from build123d import *

# Parameters (mm, degrees)
SKETCH2_W               = 121
SKETCH2_H               = 180
BOSS_EXTRUDE1_DEPTH     = 970
CUT_EXTRUDE1_DEPTH      = 1359.721825835
CUT_EXTRUDE1_DEPTH_BACK = 1359.721825835
CUT_EXTRUDE5_DEPTH      = 1625
SKETCH4_R               = 8.5
CUT_EXTRUDE6_DEPTH      = 78


with BuildPart() as part:
    # Sketch2 → Boss-Extrude1 (new body)
    with BuildSketch(Plane(origin=(0, 0, 0), x_dir=(1, 0, 0), z_dir=(0, 1, 0))):
        Polygon((300, -515), (800, -515), (800, 515), (300, 515), (300, 175), (-404, 175), (-525, 175), (-800, 175), (-800, -175), (300, -175), align=None)
        with Locations((-464.5, 265)):
            Rectangle(SKETCH2_W, SKETCH2_H)
    extrude(amount=BOSS_EXTRUDE1_DEPTH)

    # Sketch1 → Cut-Extrude1 (cut, two sides: drawn at the far end of the back side and taken through both)
    with BuildSketch(Plane.XY.offset(-CUT_EXTRUDE1_DEPTH_BACK)):
        Polygon((-800, 970), (530, 970), (300, 730), (-400, 600), (-800, 500), align=None)
    extrude(amount=CUT_EXTRUDE1_DEPTH + CUT_EXTRUDE1_DEPTH_BACK, mode=Mode.SUBTRACT)

    # Sketch3 → Cut-Extrude5 (cut)
    with BuildSketch(Plane.ZY.offset(800)):
        with BuildLine():
            Line((-165, 100), (-165, 20))
            ThreePointArc((-165, 20), (-162.071067812, 12.928932188), (-155, 10))
            Line((-155, 10), (-75, 10))
            ThreePointArc((-75, 10), (-67.928932188, 12.928932188), (-65, 20))
            Line((-65, 20), (-65, 100))
            ThreePointArc((-65, 100), (-67.928932188, 107.071067812), (-75, 110))
            Line((-75, 110), (-155, 110))
            ThreePointArc((-155, 110), (-162.071067812, 107.071067812), (-165, 100))
        make_face()
        with BuildLine():
            Line((75, 110), (155, 110))
            ThreePointArc((155, 110), (162.071067812, 107.071067812), (165, 100))
            Line((165, 100), (165, 20))
            ThreePointArc((165, 20), (162.071067812, 12.928932188), (155, 10))
            Line((155, 10), (75, 10))
            ThreePointArc((75, 10), (67.928932188, 12.928932188), (65, 20))
            Line((65, 20), (65, 100))
            ThreePointArc((65, 100), (67.928932188, 107.071067812), (75, 110))
        make_face()
    extrude(amount=-CUT_EXTRUDE5_DEPTH, mode=Mode.SUBTRACT)

    # Sketch4 → Cut-Extrude6 (cut)
    with BuildSketch(Plane.XZ):
        with Locations(Location((-498.5, 115, 0), (0, 0, 270))):
            Circle(SKETCH4_R)
        with Locations(Location((-501, -115, 0), (0, 0, 270))):
            Circle(SKETCH4_R)
        with Locations(Location((501, -115, 0), (0, 0, 270))):
            Circle(SKETCH4_R)
        with Locations(Location((498.5, 115, 0), (0, 0, 90))):
            Circle(SKETCH4_R)
    extrude(amount=-CUT_EXTRUDE6_DEPTH, mode=Mode.SUBTRACT)


solid = part.part
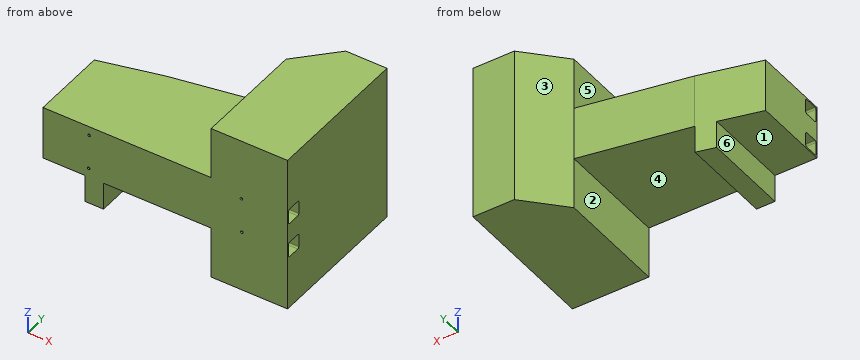
Design review of the part built by this model. Coordinates are the model's own, in mm. Face numbers are marked on the shaded views. A direction names the side the tool comes from. Round coordinates to 2 decimals unless told otherwise and drop trailing zeros. Write each loop counter-clockwise with the first axis right and the second up, starting at its lowest first coordinate (ties: lowest second). Pieces come first, ordered by that corner, then holes. Notation, with made-up numbers: (51.5, -1.75) -> (109.5, -1.75) arc R23 ccw to (109.5, 25.25) -> close; hole circle Ø1 at (22, 77). An arc over 180 degrees is marked (long way). One line per item, written item: value. Start each with the question number.
Q1. Insertion check: P1, Ø15.5, axis at x = 498.5, z = 115, coming from the +Y side; P2, Ø6, axis at x = -502.5, y = 113, coming from the +Z side; P3, Ø2, axis at x = 3.5, y = 564.5, coming from the -Z side. Each pin has a flat end and moves straight along its axis. Give the tip position at first contact, or say it passes through.
Q2. Add section A-A (x = 687). Give the boundary of the cut face in (y, z).
Q3. Tool access review of the marked faces 4, 5 and 6: name each direction out of +Z, -Z, +X, -X, +Y, -Y from which nothing blocks a thin tool from reaching the whole face with its end or side.
Q4. To check wall thickness, follow probe 1 along X at (y, z) = (5.75, 115); probe 2 along X at (y, z) = (3, -115); probe 3 along Z at (x, y) = (277, 82). State the ranges of each line that lie inside material, in increasing order.
Q5. The part is to be moulded in two halves that separate along X. For the marked faces 1, 2 and 3, say which applies: pulls with the +X half, pulls with the -X half, needs draft (parallel to the pull), parting line crosses it, or undercut.
Q6. Add section B-B (z = 15.5). Give the boundary of the cut face in (x, y), then the cut area to 3 significant figures.
Q7. Add section D-D (x = -621). Give the boundary of the cut face in (y, z), then the cut area to 3 significant figures.
Q8. Add section C-C (y = 379). Give the boundary of the cut face in (x, z), then the cut area to 3 significant figures.
Response:
1. P1: stops at y = 945.22
1. P2: stops at z = 175
1. P3: stops at z = -175
2. outline: (0, -515) -> (970, -515) -> (970, 515) -> (0, 515) -> close; hole (10, -155) arc R10 ccw to (20, -165) -> (100, -165) arc R10 ccw to (110, -155) -> (110, -75) arc R10 ccw to (100, -65) -> (20, -65) arc R10 ccw to (10, -75) -> close; hole (10, 75) arc R10 ccw to (20, 65) -> (100, 65) arc R10 ccw to (110, 75) -> (110, 155) arc R10 ccw to (100, 165) -> (20, 165) arc R10 ccw to (10, 155) -> close
3. face 4: -Z, +Y, -Y
3. face 5: +Z, -X, +Y, -Y
3. face 6: -Z, -X, +Y, -Y
4. probe 1: x = -800 to -507, -490 to 490, 507 to 800
4. probe 2: x = -800 to -509.5, -492.5 to 492.5, 509.5 to 800
4. probe 3: z = -175 to -165, -65 to 65, 165 to 175
5. face 1: needs draft
5. face 2: undercut
5. face 3: pulls with the -X half
6. outline: (-800, 0) -> (800, 0) -> (800, 970) -> (530, 970) -> (300, 730) -> (-400, 600) -> (-800, 500) -> close
6. area: 1,140,000 mm^2
7. outline: (0, -175) -> (544.75, -175) -> (544.75, 175) -> (0, 175) -> close; hole (10, -155) arc R10 ccw to (20, -165) -> (100, -165) arc R10 ccw to (110, -155) -> (110, -75) arc R10 ccw to (100, -65) -> (20, -65) arc R10 ccw to (10, -75) -> close; hole (10, 75) arc R10 ccw to (20, 65) -> (100, 65) arc R10 ccw to (110, 75) -> (110, 155) arc R10 ccw to (100, 165) -> (20, 165) arc R10 ccw to (10, 155) -> close
7. area: 171,000 mm^2
8. outline: (-800, -175) -> (-525, -175) -> (-525, -355) -> (-404, -355) -> (-404, -175) -> (300, -175) -> (300, -515) -> (800, -515) -> (800, 515) -> (300, 515) -> (300, 175) -> (-800, 175) -> close
8. area: 922,000 mm^2
